Model file for the job. Use its own axes, mm. Face numbers are marked on the shaded views. A direction names the side the tool comes from. Coordinates: 2 decimals unless noted, no trailing zeros. Order: outer loops, then holes, each group sorted by start corner. A loop starts at its lowest first (then second) coordinate and runs counter-clockwise, first axis right, second up.
from build123d import *

# Parameters (mm, degrees)
F1_DEPTH = 8.5
F2_R     = 5.08
F3_DEPTH = 10.8966
F4_SIZE  = 2


# Not quite as in the source:
# - a feature of the source that left no trace in its solid (it failed there, or was rolled back) is left out


with BuildPart() as f1:
    # F0 (on Top) → F1 (new body)
    with BuildSketch(Plane.XY):
        with BuildLine():
            Line((8.9732294485, 7.7602798555), (-3.8267705515, 7.7602798555))
            Line((-3.8267705515, 7.7602798555), (-3.8267705515, -8.2397201445))
            ThreePointArc((-3.8267705515, -8.2397201445), (-0.2330190264, 2.0052786354), (8.9732294485, 7.7602798555))
        make_face()
        with BuildLine():
            Line((16.1732294485, 7.7602798555), (8.9732294485, 7.7602798555))
            ThreePointArc((8.9732294485, 7.7602798555), (-0.2330190264, 2.0052786354), (-3.8267705515, -8.2397201445))
            Line((-3.8267705515, -8.2397201445), (16.1732294485, -8.2397201445))
            Line((16.1732294485, -8.2397201445), (16.1732294485, 7.7602798555))
        make_face()
    extrude(amount=F1_DEPTH)

    # F2
    f2_edges = [f1.edges().sort_by_distance(p)[0] for p in [
        (16.173229, -0.23972, 8.5),
        (6.173229, -8.23972, 8.5),
    ]]
    fillet(f2_edges, radius=F2_R)

    # F3 (add): a face of the model
    f3_faces = [f1.faces().sort_by_distance(p)[0] for p in [
        (6.1732294485, -8.2397201445, 1.71),
    ]]
    extrude(f3_faces, amount=F3_DEPTH)

    # F4
    f4_edges = [f1.edges().sort_by_distance(p)[0] for p in [
        (16.173229, -13.68802, 3.42),
        (6.173229, -19.13632, 3.42),
    ]]
    chamfer(f4_edges, length=F4_SIZE)


solid = f1.part
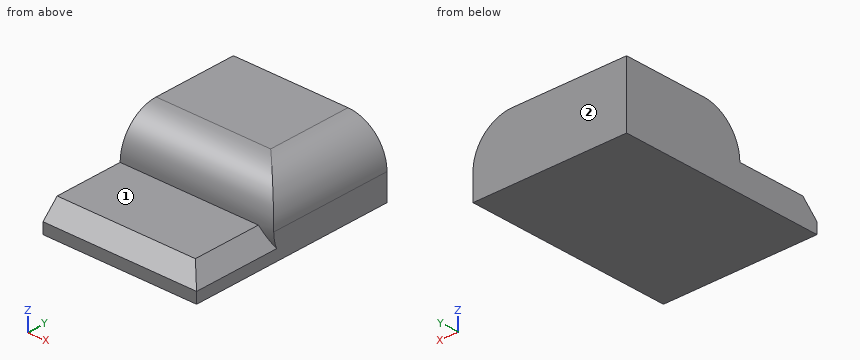
Q1. Cut at D-D, the plane x = 6.5. List the corners of the cut face in (y, z).
Established:
outline: (-19.14, 0) - (7.76, 0) - (7.76, 8.5) - (-3.16, 8.5) arc R5.08 ccw to (-8.24, 3.42) - (-17.14, 3.42) - (-19.14, 1.42) - close
Q2. Cut at A-A, the plane y = -0.5. List the corners of the cut face in (x, z).
Established:
outline: (-3.83, 0) - (16.17, 0) - (16.17, 3.42) arc R5.08 ccw to (11.09, 8.5) - (-3.83, 8.5) - close
Q3. Probe line 1 (Z direction, x = 5, y = -10.25); line 2 (Y direction, x = 2.75, z = 4.25); line 3 (X direction, y = 2, z = 7.5). List the from-to ranges inside material, lowest first.
Established:
line 1: z = 0 to 3.42
line 2: y = -8.17 to 7.76
line 3: x = -3.83 to 14.12
Q4. Cut at B-B, the plane x = 13.25. List the corners of the cut face in (y, z).
Established:
outline: (-19.14, 0) - (7.76, 0) - (7.76, 8.02) - (-5.32, 8.02) arc R5.08 ccw to (-8.24, 3.42) - (-17.14, 3.42) - (-19.14, 1.42) - close
Q5. Drop a flat-ended pin along its axis: P1, Ø10, axis at x = 1, y = -12.5, coming from the +Z side. Give the stop position or say it passes through.
Established:
P1: stops at z = 6.06
Q6. Which spindle directions (+Z, -Z, +X, -X, +Y, -Y) get a long thin tool onto all of the face, cutting with end or side? Do the marked faces 1 and 2. Say none if no direction does.
Established:
face 1: +Z, +X, -X, -Y
face 2: +Z, -Z, +X, -X, +Y
Q7. Cut at C-C, the plane z = 2.25. List the corners of the cut face in (x, y).
Established:
outline: (-3.83, -18.31) - (15.34, -18.31) - (15.34, -8.1) - (16.17, -8.1) - (16.17, 7.76) - (-3.83, 7.76) - close
